Work out the finished part from the listing and answer in its coordinate system (mm). Face numbers are marked on the shaded views. Give positions to 0.01 mm unless a question says otherwise; leave off trailing zeros. Order: outer loops, then holes, each group sorted by start corner. A loop starts at its lowest first (then second) coordinate and runs counter-clockwise, first axis right, second up. Notation, with made-up numbers: (80, -3) -> (138, -3) arc R19 ccw to (138, 23) -> close; hole circle Ø3 at (-10.75, -26). An arc over 180 degrees is marked (long way). Use a Markdown table: item, result. Add a question column.
```python
from build123d import *

# Parameters (mm, degrees)
SKETCH2_R                      = 38.75
BOSS_EXTRUDE1_DEPTH            = 8.8
BOSS_EXTRUDE2_DEPTH            = 9.8
BOSS_EXTRUDE2_DEPTH_BACK       = 9.8
CUT_EXTRUDE1_REACH             = 48.75
CUT_EXTRUDE1_DIRECTION_2_REACH = 48.75
CUT_EXTRUDE2_REACH             = 48.75
SKETCH5_W                      = 2
SKETCH5_H                      = 1


with BuildPart() as part:
    # Sketch2 → Boss-Extrude1 (new body)
    with BuildSketch(Plane(origin=(0, 0, 0), x_dir=(1, 0, 0), z_dir=(0, 1, 0))):
        with BuildLine():
            Line((-11.788704897, -9.8), (0, -9.8))
            Line((0, -9.8), (0, 9.8))
            Line((0, 9.8), (-11.788704897, 9.8))
            ThreePointArc((-11.788704897, 9.8), (-104.25, 0), (-11.788704897, -9.8))
        make_face()
        with Locations((-57.5, 0)):
            Circle(SKETCH2_R, mode=Mode.SUBTRACT)
    extrude(amount=-BOSS_EXTRUDE1_DEPTH)

    # Sketch3 → Boss-Extrude2 (add, two sides)
    with BuildSketch(Plane.XY) as boss_extrude2_sk:
        with BuildLine():
            Line((0, -8.8), (0, 0))
            Line((0, 0), (-17.6, 0))
            Line((-17.6, 0), (-4.4, 7.621023553))
            ThreePointArc((-4.4, 7.621023553), (8.500147271, 2.277607597), (0, -8.8))
        make_face()
    extrude(amount=BOSS_EXTRUDE2_DEPTH)
    extrude(boss_extrude2_sk.sketch, amount=-BOSS_EXTRUDE2_DEPTH_BACK)

    # Sketch4 → Cut-Extrude1 (cut, up to next)
    with BuildSketch(Plane.XY, mode=Mode.PRIVATE) as cut_extrude1_sk1:
        Polygon((5.773502692, 0), (2.886751346, 5), (-2.886751346, 5), (-5.773502692, 0), (-2.886751346, -5), (2.886751346, -5), align=None)
    cut_extrude1_tool1 = extrude(cut_extrude1_sk1.sketch, amount=-CUT_EXTRUDE1_REACH, mode=Mode.PRIVATE) & part.part
    add(cut_extrude1_tool1.solids().sort_by_distance((0, 0, 0))[0], mode=Mode.SUBTRACT)

    # Sketch4 → Cut-Extrude1 direction 2 (cut, up to next)
    with BuildSketch(Plane.XY, mode=Mode.PRIVATE) as cut_extrude1_direction_2_sk1:
        Polygon((5.773502692, 0), (2.886751346, 5), (-2.886751346, 5), (-5.773502692, 0), (-2.886751346, -5), (2.886751346, -5), align=None)
    cut_extrude1_direction_2_tool1 = extrude(cut_extrude1_direction_2_sk1.sketch, amount=CUT_EXTRUDE1_DIRECTION_2_REACH, mode=Mode.PRIVATE) & part.part
    add(cut_extrude1_direction_2_tool1.solids().sort_by_distance((0, 0, 0))[0], mode=Mode.SUBTRACT)

    # Sketch5 → Cut-Extrude2 (cut, up to next)
    with BuildSketch(Plane.XY, mode=Mode.PRIVATE) as cut_extrude2_sk1:
        with Locations((0, -5.5)):
            Rectangle(SKETCH5_W, SKETCH5_H)
    cut_extrude2_tool1 = extrude(cut_extrude2_sk1.sketch, amount=-CUT_EXTRUDE2_REACH, mode=Mode.PRIVATE) & part.part
    add(cut_extrude2_tool1.solids().sort_by_distance((0, -5.5, 0))[0], mode=Mode.SUBTRACT)


solid = part.part
```
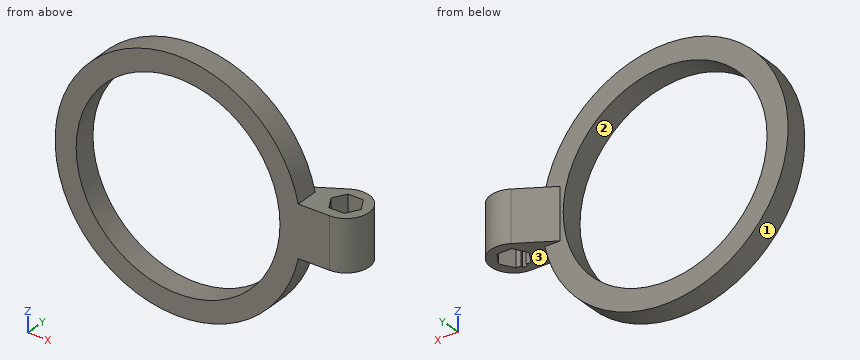
1) Determine the mould class of the marked faces 1, 2 and 3 for opening direction Z: released by +Z, released by -Z, zero draft, split by the parting line, or undercut.
2) The part is cut by section A-A, the plane x = -57.5. Determine the outline of the cut face in (y, z).
3) The part is cut by section B-B, the plane z = 34.5. Determine the outline of the cut face in (x, y), then the cut area to 3 significant figures.
4) Flat-ended cylindrical pins translate along their axes: pin 1 (8 mm diameter, centred on x = -27, z = -30, fed in from +Y); pin 2 (2 mm diameter, centred on y = -5, z = 6.5, fed in from +X); pin 3 (0.8 mm diameter, centred on y = -5.5, z = -2.5, fed in from +X); pin 4 (10 mm diameter, centred on x = -43, z = 26, fed in from -Y). Find the tip coordinate at first contact, or state that the pin passes through.
5) Straight lines are drawn through the part: line 1 (Z direction, x = -57.5, y = -4.5); line 2 (X direction, y = -3, z = 0); line 3 (X direction, y = -3.25, z = 0). For each, find the intervals that lie inside material, in ascending order.
A:
| question | item | result |
|---|---|---|
| 1 | face 1 | split by the parting line |
| 1 | face 2 | undercut |
| 1 | face 3 | released by -Z |
| 2 | outline | (-8.8, -46.75) -> (0, -46.75) -> (0, -38.75) -> (-8.8, -38.75) -> close; (-8.8, 38.75) -> (0, 38.75) -> (0, 46.75) -> (-8.8, 46.75) -> close |
| 3 | outline | (-89.05, -8.8) -> (-75.14, -8.8) -> (-75.14, 0) -> (-89.05, 0) -> close; (-39.86, -8.8) -> (-25.95, -8.8) -> (-25.95, 0) -> (-39.86, 0) -> close |
| 3 | area | 245 mm^2 |
| 4 | pin 1 | y = 0 |
| 4 | pin 2 | x = 7.84 |
| 4 | pin 3 | x = 7.17 |
| 4 | pin 4 | through |
| 5 | line 1 | -46.75 to -38.75, 38.75 to 46.75 |
| 5 | line 2 | -104.25 to -96.25, -18.75 to -4.04, 4.04 to 8.27 |
| 5 | line 3 | -104.25 to -96.25, -18.75 to -3.9, 3.9 to 8.18 |
